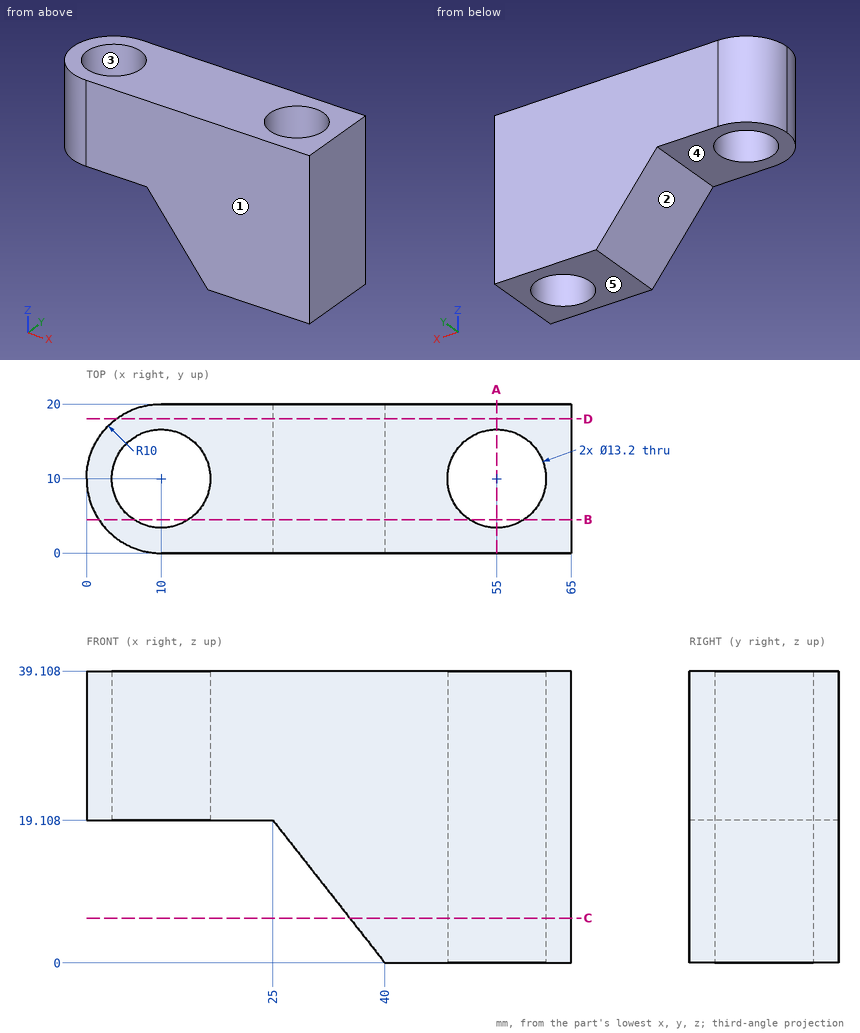
Here's the drawing with two shaded views (mm, measured from the low corner). I have some questions. A direction names the side the tool comes from. Round coordinates to 2 decimals unless told otherwise and drop trailing zeros. Order: outer loops, then holes, each group sorted by start corner. A loop starts at its lowest first (then second) coordinate and runs counter-clockwise, first axis right, second up. Notation, with made-up numbers: (44.25, 82.25) -> (48.25, 82.25) arc R26 ccw to (48.25, 103.25) -> close; hole circle Ø8 at (-31.75, 25). An arc over 180 degrees is marked (long way). Return JSON: item names as keys, results as strings.
Q1. If we section it at A-A on x = 55: List the corners of the cut face in (y, z) for me.
Filled sheet:
{"outline": "(0, 0) -> (3.4, 0) -> (3.4, 39.11) -> (0, 39.11) -> close; (16.6, 0) -> (20, 0) -> (20, 39.11) -> (16.6, 39.11) -> close"}
Q2. Which directions (+Z, -Z, +X, -X, +Y, -Y) give clear straight access to the entire face, cutting with the end or side of a thin tool? Please do the marked faces 4 and 5.
Filled sheet:
{"face 4": "-Z, -X, +Y, -Y", "face 5": "-Z, +X, -X, +Y, -Y"}
Q3. If we section it at C-C on z = 6: List the corners of the cut face in (x, y) for me, plus the area to 3 significant figures.
Filled sheet:
{"outline": "(35.29, 0) -> (65, 0) -> (65, 20) -> (35.29, 20) -> close; hole circle Ø13.2 at (55, 10)", "area": "457 mm^2"}
Q4. For pin 1 Ø10 at (x, y) = (6.5, 6.5) entering from -Z; pin 2 Ø5 at (y, z) = (15, 14) entering from -X; pin 3 Ø5 at (y, z) = (2.5, 26) entering from -X, each with a flat end and sliding along its axis, tell me the tip position at first contact or that it passes through.
Filled sheet:
{"pin 1": "stops at z = 19.11", "pin 2": "stops at x = 27.05", "pin 3": "stops at x = 1.34"}
Q5. If we section it at B-B on y = 4.5: List the corners of the cut face in (x, z) for me, plus the area to 3 significant figures.
Filled sheet:
{"outline": "(1.65, 19.11) -> (6.35, 19.11) -> (6.35, 39.11) -> (1.65, 39.11) -> close; (13.65, 19.11) -> (25, 19.11) -> (40, 0) -> (51.35, 0) -> (51.35, 39.11) -> (13.65, 39.11) -> close; (58.65, 0) -> (65, 0) -> (65, 39.11) -> (58.65, 39.11) -> close", "area": "1,460 mm^2"}
Q6. I need wall thicknesses on line 1 along X through (y, z) = (8, 36.5); line 2 along X through (y, z) = (11.75, 32) (1 decimal); line 3 along Y through (x, z) = (55, 20). Which ranges of each line are inside material? Lowest first, please. Write a range as from..to.
Filled sheet:
{"line 1": "x = 0.2..3.71, 16.29..48.71, 61.29..65", "line 2": "x = 0.2..3.6, 16.4..48.6, 61.4..65", "line 3": "y = 0..3.4, 16.6..20"}
Q7. If we section it at D-D on y = 18: List the corners of the cut face in (x, z) for me, plus the area to 3 significant figures.
Filled sheet:
{"outline": "(4, 19.11) -> (25, 19.11) -> (40, 0) -> (65, 0) -> (65, 39.11) -> (4, 39.11) -> close", "area": "1,840 mm^2"}
Q8. If we mould it in two halves opening along Y, with no side actions, what happens to the marked faces 1, 2 and 3? For each: released by +Y, released by -Y, zero draft, split by the parting line, or undercut.
Filled sheet:
{"face 1": "released by -Y", "face 2": "zero draft", "face 3": "undercut"}
